from build123d import *

# Parameters (mm, degrees)
EXTRUDE_1_DEPTH = 32
FILLET_1_R      = 1
SHELL_2_T       = -2


with BuildPart() as part:
    # Эскиз1 → Бобышка-Вытянуть1 (new body)
    with BuildSketch(Plane(origin=(0, 0, 0), x_dir=(1, 0, 0), z_dir=(0, 1, 0))):
        with BuildLine():
            Line((-7, 0), (-76, 0))
            ThreePointArc((-76, 0), (-80.949747468, 2.050252532), (-83, 7))
            Line((-83, 7), (-83, 175))
            ThreePointArc((-83, 175), (-80.949747468, 179.949747468), (-76, 182))
            Line((-76, 182), (-7, 182))
            ThreePointArc((-7, 182), (-2.050252532, 179.949747468), (0, 175))
            Line((0, 175), (0, 7))
            ThreePointArc((0, 7), (-2.050252532, 2.050252532), (-7, 0))
        make_face()
    extrude(amount=EXTRUDE_1_DEPTH)

    # Скругление1
    fillet_1_edges = [part.edges().sort_by_distance(p)[0] for p in [
        (0, 0, -91),
        (-2.050252532, 0, -2.050252532),
        (-41.5, 0, 0),
        (-80.949747468, 0, -2.050252532),
        (-83, 0, -91),
        (-80.949747468, 0, -179.949747468),
        (-41.5, 0, -182),
        (-2.050252532, 0, -179.949747468),
    ]]
    fillet(fillet_1_edges, radius=FILLET_1_R)

    # Оболочка2
    shell_2_openings = [part.faces().sort_by_distance(p)[0] for p in [
        (-41.5, 32, -91),
    ]]
    offset(amount=SHELL_2_T, openings=shell_2_openings, kind=Kind.INTERSECTION)


solid = part.part
Can you work these out from the model? Positions are in its coordinate system, mm. A direction names the side the tool comes from. Give positions to 0.01 mm unless a question says otherwise; leave off trailing zeros. Order: outer loops, then holes, each group sorted by start corner. A loop starts at its lowest first (then second) coordinate and runs counter-clockwise, first axis right, second up. Notation, with made-up numbers: M 39.5,-8 L 61.5,-8 A17 cw 61.5,24 Z; hole C -38.5,11.25 d8. An arc over 180 degrees is marked long. Use one line per item in the form item = value. Start each with the question number.
Item 1: If we section it at C-C (x = -45): Write out the boundary of the cut face in (y, z), then the cut area to 3 significant figures.
Item 2: If we section it at A-A (y = 7.5): Write out the boundary of the cut face in (x, z).
Item 3: We'd pull the mould along X, two halves only. Please class faces 3 (the cylindrical face through (-2, 16.3, -2.1)), 4 (the flat face through (-81, 17, -90)), 5 (the flat face through (-83, 16, -90)): +X half, -X half, draft (parallel to the pull), parting line (faces both ways), or undercut.
Item 4: Will this pin go through, and if not, where does the flat tip stop? pin 1 Ø23.5 at (x, z) = (-44.5, -85.5) entering from +Y.
Item 5: For faces 1 (the flat face through (-2, 17, -92)), 2 (the flat face through (0, 16, -92)), which set-ups out of +Z, -Z, +X, -X, +Y, -Y let a thin tool reach every point of the face, with its end or its side?
Item 6: If we section it at B-B (z = -96): Write out the boundary of the cut face in (x, y).
Item 7: If I drill on line 1 along X through (y, z) = (20, -54); line 2 along Z through (x, y) = (-50, 19.5); line 3 along Y through (x, z) = (-57, -143.5), over which ranges is the centre line in solid material (lowest first)?
Outcome:
q1.outline = M 0,-181 A1 ccw 1,-182 L 32,-182 L 32,-180 L 2,-180 L 2,-2 L 32,-2 L 32,0 L 1,0 A1 ccw 0,-1 Z
q1.area = 484 mm2
q2.outline = M -83,-175 A7 ccw -76,-182 L -7,-182 A7 ccw 0,-175 L 0,-7 A7 ccw -7,0 L -76,0 A7 ccw -83,-7 Z; hole M -81,-175 A5 ccw -76,-180 L -7,-180 A5 ccw -2,-175 L -2,-7 A5 ccw -7,-2 L -76,-2 A5 ccw -81,-7 Z
q3.face_3 = +X half
q3.face_4 = undercut
q3.face_5 = -X half
q4.pin_1 = 2
q5.face_1 = +Y
q5.face_2 = +Z, -Z, +X, +Y, -Y
q6.outline = M -83,1 A1 ccw -82,0 L -1,0 A1 ccw 0,1 L 0,32 L -2,32 L -2,2 L -81,2 L -81,32 L -83,32 Z
q7.line_1 = -83 to -81, -2 to 0
q7.line_2 = -182 to -180, -2 to 0
q7.line_3 = 0 to 2
